Geometry: final body of the model. Coordinates: model frame, mm. Face numbers are marked on the shaded views. A direction names the side the tool comes from. Round coordinates to 2 decimals unless told otherwise and drop trailing zeros. Loops run counter-clockwise (first coordinate to the right, second up) from the corner with the lowest first, then second, coordinate; pieces in that order, holes last. Notation, with made-up numbers: (85, 78) -> (98, 78) arc R20 cw to (98, 102) -> close; hole circle Ø1 at (-25, 74). An arc over 180 degrees is marked (long way). Answer in a Markdown table with one row per item.
```python
from build123d import *

# Parameters (mm, degrees)
F1_DEPTH = 25.4
F3_DEPTH = 30.734
F4_W     = 10.16
F4_H     = 6.604
F5_DEPTH = 51.463376
F6_W     = 10.16
F6_H     = 6.604
F7_DEPTH = 51.463376


with BuildPart() as f1:
    # F0 (on Top) → F1 (new body)
    with BuildSketch(Plane.XY):
        with BuildLine():
            Line((27.759297, 87.433918), (-30.660703, 87.433918))
            Line((-30.660703, 87.433918), (-30.660703, -17.214082))
            Line((-30.660703, -17.214082), (-23.040703, -64.868706))
            Line((-23.040703, -64.868706), (-11.356703, -64.868706))
            Line((-11.356703, -64.868706), (-11.356703, -36.420706))
            ThreePointArc((-11.356703, -36.420706), (-1.450703, -26.514706), (8.455297, -36.420706))
            Line((8.455297, -36.420706), (8.455297, -64.868706))
            Line((8.455297, -64.868706), (20.139297, -64.868706))
            Line((20.139297, -64.868706), (27.759297, -17.214082))
            Line((27.759297, -17.214082), (27.759297, 87.433918))
        make_face()
    extrude(amount=F1_DEPTH)

    # F2 (on face) → F3 (join)
    with BuildSketch(Plane(origin=(0, 87.433918, 0), x_dir=(-1, 0, 0), z_dir=(0, 1, 0))):
        Polygon((10.477128, 51.462376), (-7.575722, 51.462376), (-27.759297, 39.809384), (-27.759297, 25.4), (30.660703, 25.4), (30.660703, 39.809384), align=None)
    extrude(amount=-F3_DEPTH)

    # F4 (on face) → F5 (cut, through all)
    with BuildSketch(Plane(origin=(0, 0, 0), x_dir=(1, 0, 0), z_dir=(0, 0, -1))):
        with Locations((-25.580703, -84.131918)):
            Rectangle(F4_W, F4_H)
    extrude(amount=-F5_DEPTH, mode=Mode.SUBTRACT)

    # F6 (on face) → F7 (cut, through all)
    with BuildSketch(Plane(origin=(0, 0, 0), x_dir=(1, 0, 0), z_dir=(0, 0, -1))):
        with Locations((22.679297, -84.131918)):
            Rectangle(F6_W, F6_H)
    extrude(amount=-F7_DEPTH, mode=Mode.SUBTRACT)


solid = f1.part
```
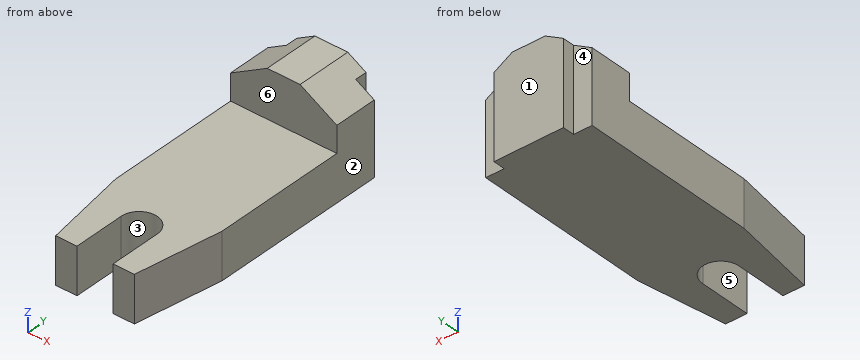
Item 1: Reachability of the marked faces 4, 5 and 6 from +Z, -Z, +X, -X, +Y, -Y: full face, straight path, thin tool, end or side. Return the list, or none.
Answer:
| item | result |
|---|---|
| face 4 | +Z, -Z, -X, +Y |
| face 5 | +Z, -Z, -Y |
| face 6 | +Z, +X, -X, -Y |
Item 2: Cut plane C-C (x = 3). Output: boundary loops of the cut face in (y, z).
Answer:
| item | result |
|---|---|
| outline | (-27.57, 0) -> (87.43, 0) -> (87.43, 51.46) -> (56.7, 51.46) -> (56.7, 25.4) -> (-27.57, 25.4) -> close |
Item 3: Cut plane A-A (z = 36.5). Output: boundary loops of the cut face in (x, y), then the cut area to 3 significant figures.
Answer:
| item | result |
|---|---|
| outline | (-30.66, 56.7) -> (27.76, 56.7) -> (27.76, 80.83) -> (17.6, 80.83) -> (17.6, 87.43) -> (-20.5, 87.43) -> (-20.5, 80.83) -> (-30.66, 80.83) -> close |
| area | 1,660 mm² |
Item 4: Cut plane B-B (y = 63.5). Output: boundary loops of the cut face in (x, z), then the cut area to 3 significant figures.
Answer:
| item | result |
|---|---|
| outline | (-30.66, 0) -> (27.76, 0) -> (27.76, 39.81) -> (7.58, 51.46) -> (-10.48, 51.46) -> (-30.66, 39.81) -> close |
| area | 2,770 mm² |
Item 5: Pin query (flat end, axial travel): pin 1 Ø8 at (x, z) = (14, 35.5) entering from -Y; pin 2 Ø10 at (x, y) = (-18.5, -21.5) entering from +Z; pin 3 Ø7.5 at (y, z) = (-48, 15.5) entering from -X. Return the tip coordinate at first contact, or that it passes through.
Answer:
| item | result |
|---|---|
| pin 1 | stops at y = 56.7 |
| pin 2 | stops at z = 25.4 |
| pin 3 | stops at x = -26.34 |
Item 6: Cut plane D-D (z = 23.5). Output: boundary loops of the cut face in (x, y).
Answer:
| item | result |
|---|---|
| outline | (-30.66, -17.21) -> (-23.04, -64.87) -> (-11.36, -64.87) -> (-11.36, -36.42) arc R9.91 cw to (8.46, -36.42) -> (8.46, -64.87) -> (20.14, -64.87) -> (27.76, -17.21) -> (27.76, 80.83) -> (17.6, 80.83) -> (17.6, 87.43) -> (-20.5, 87.43) -> (-20.5, 80.83) -> (-30.66, 80.83) -> close |
Item 7: Line query: probe 1 along Z at (x, y) = (-23, 6); probe 2 along Y at (x, z) = (0.5, 46.5); probe 3 along Y at (x, z) = (20.5, 41.5). Output: solid intervals per line, ascending. Write a range as [from, to].
Answer:
| item | result |
|---|---|
| probe 1 | z = [0, 25.4] |
| probe 2 | y = [56.7, 87.43] |
| probe 3 | y = [56.7, 80.83] |
Item 8: Draft query along X for the marked faces 1, 2 and 3. Return one class per face: pulls with the +X half, pulls with the -X half, needs draft (parallel to the pull), parting line crosses it, or undercut.
Answer:
| item | result |
|---|---|
| face 1 | needs draft |
| face 2 | pulls with the +X half |
| face 3 | undercut |
